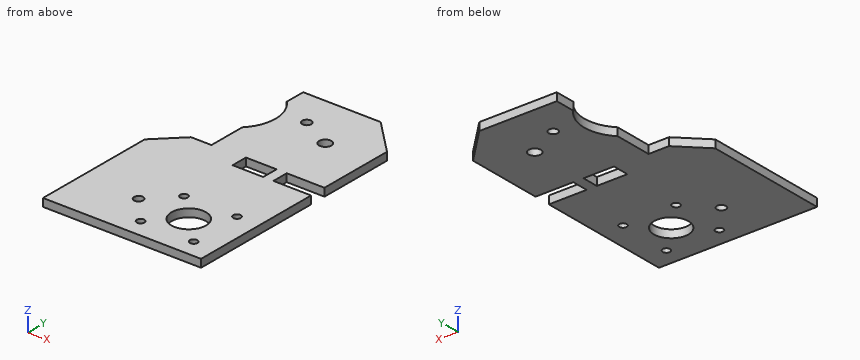
```python
from build123d import *

# Parameters (mm, degrees)
SKETCH1_W            = 155
SKETCH1_H            = 257
BOSS_EXTRUDE1_DEPTH  = 7.7
CHAMFER1_SIZE        = 34
SKETCH2_R            = 4.5
SKETCH2_W            = 37
SKETCH2_H            = 16
CUT_EXTRUDE1_DEPTH   = 10
SKETCH3_R            = 38.109899267
CUT_EXTRUDE2_DEPTH   = 10
CUT_EXTRUDE3_DEPTH   = 10
SKETCH5_R            = 16.935062279
CUT_EXTRUDE4_DEPTH   = 10
SKETCH6_R            = 3.705491154
CUT_EXTRUDE5_DEPTH   = 10
LPATTERN1_COUNT      = 2
LPATTERN1_PITCH      = 52
LPATTERN1_COUNT_DIR2 = 2
LPATTERN1_PITCH_DIR2 = 52
SKETCH7_R            = 6
CUT_EXTRUDE6_DEPTH   = 10
SKETCH8_W            = 30
SKETCH8_H            = 16
CUT_EXTRUDE7_DEPTH   = 10


with BuildPart() as part:
    # Sketch1 → Boss-Extrude1 (new body)
    with BuildSketch(Plane.XY):
        with Locations((64.176783005, -115.237481032)):
            Rectangle(SKETCH1_W, SKETCH1_H)
    extrude(amount=BOSS_EXTRUDE1_DEPTH)

    # Chamfer1
    chamfer1_edges = [part.edges().sort_by_distance(p)[0] for p in [
        (141.676783005, 13.262518968, 3.85),
    ]]
    chamfer(chamfer1_edges, length=CHAMFER1_SIZE)

    # Sketch2 → Cut-Extrude1 (cut)
    with BuildSketch(Plane.XY.offset(7.7)):
        with Locations((64.676783005, -22.737481032)):
            Circle(SKETCH2_R)
        with Locations((43.676783005, -198.737481032)):
            Circle(SKETCH2_R)
        with Locations((123.176783005, -103.737481032)):
            Rectangle(SKETCH2_W, SKETCH2_H)
    extrude(amount=-CUT_EXTRUDE1_DEPTH, mode=Mode.SUBTRACT)

    # Sketch3 → Cut-Extrude2 (cut)
    with BuildSketch(Plane.XY.offset(7.7)):
        with Locations((4.429117296, -33.119350325)):
            Circle(SKETCH3_R)
    extrude(amount=-CUT_EXTRUDE2_DEPTH, mode=Mode.SUBTRACT)

    # Sketch4 → Cut-Extrude3 (cut)
    with BuildSketch(Plane.XY.offset(7.7)):
        Polygon((31.676783005, 13.262518968), (31.676783005, -96.737481032), (11.676783005, -96.737481032), (-13.323216995, -121.737481032), (-67.69781948, -122.43585218), (-69.553853122, 22.073398829), (23.898503121, 29.809405578), align=None)
    extrude(amount=-CUT_EXTRUDE3_DEPTH, mode=Mode.SUBTRACT)

    # Sketch5 → Cut-Extrude4 (cut)
    with BuildSketch(Plane.XY.offset(7.7)):
        with Locations((93.676783005, -199.737481032)):
            Circle(SKETCH5_R)
    extrude(amount=-CUT_EXTRUDE4_DEPTH, mode=Mode.SUBTRACT)

    # Sketch6 → Cut-Extrude5 (cut)
    with BuildSketch(Plane.XY.offset(7.7)):
        with Locations((67.676783005, -225.737481032)):
            Circle(SKETCH6_R)
    cut_extrude5 = extrude(amount=-CUT_EXTRUDE5_DEPTH, mode=Mode.SUBTRACT)

    # LPattern1: Cut-Extrude5 2 × 2
    with Locations(*[(j * LPATTERN1_PITCH_DIR2, i * LPATTERN1_PITCH, 0) for i in range(LPATTERN1_COUNT) for j in range(LPATTERN1_COUNT_DIR2) if (i, j) != (0, 0)]):
        add(cut_extrude5, mode=Mode.SUBTRACT)

    # Sketch7 → Cut-Extrude6 (cut)
    with BuildSketch(Plane.XY.offset(7.7)):
        with Locations((96.676783005, -39.737481032)):
            Circle(SKETCH7_R)
    extrude(amount=-CUT_EXTRUDE6_DEPTH, mode=Mode.SUBTRACT)

    # Sketch8 → Cut-Extrude7 (cut)
    with BuildSketch(Plane.XY.offset(7.7)):
        with Locations((79.676783005, -103.737481032)):
            Rectangle(SKETCH8_W, SKETCH8_H)
    extrude(amount=-CUT_EXTRUDE7_DEPTH, mode=Mode.SUBTRACT)


solid = part.part
```
Geometry: final body of the model. Coordinates: model frame, mm. Coordinates: 2 decimals unless noted, no trailing zeros. Loops run counter-clockwise (first coordinate to the right, second up) from the corner with the lowest first, then second, coordinate; pieces in that order, holes last. Notation, with made-up numbers: (34, 44.25) -> (81, 44.25) arc R17 ccw to (81, 56.25) -> close; hole circle Ø2 at (35, -9.75). An arc over 180 degrees is marked (long way). Use a Markdown table: item, result. Add a question column.
(1) Section query B-B, the plane z = 3.25. State how many separate pieces and enclosed holes the cut face has, plus the area to 3 significant figures.
(2) Line query: line 1 along Y through (x, z) = (72.5, 1.25); line 2 along Y through (x, z) = (123, 3); line 3 along Y through (x, z) = (101, 5.5). Output: solid intervals per line, ascending.
(3) Section query C-C, the plane x = 36. Return loops of the section in (y, z).
(4) Pin query (flat end, axial travel): pin 1 Ø10.5 at (x, y) = (64.68, -22.74) entering from +Z; pin 2 Ø1.5 at (x, z) = (116.5, 3) entering from +Y; pin 3 Ø4 at (y, z) = (-1.5, 2.5) entering from -X. Return the tip coordinate at first contact, or that it passes through.
(5) Section query D-D, the plane x = 15. Return loops of the section in (y, z).
(6) Section query A-A, the plane x = 99.5. Return loops of the section in (y, z), plus the area to 3 significant figures.
Answer:
| question | item | result |
|---|---|---|
| 1 | separate pieces | 1 |
| 1 | enclosed holes | 9 |
| 1 | area | 31,200 mm^2 |
| 2 | line 1 | y = -243.74 to -111.74, -95.74 to 13.26 |
| 2 | line 2 | y = -243.74 to -227.38, -224.1 to -175.38, -172.1 to -111.74, -95.74 to -2.06 |
| 2 | line 3 | y = -243.74 to -215.01, -184.47 to -43.9, -35.58 to 13.26 |
| 3 | outline | (-243.74, 0) -> (-54.47, 0) -> (-54.47, 7.7) -> (-243.74, 7.7) -> close; (-11.77, 0) -> (13.26, 0) -> (13.26, 7.7) -> (-11.77, 7.7) -> close |
| 4 | pin 1 | stops at z = 7.7 |
| 4 | pin 2 | stops at y = 5.19 |
| 4 | pin 3 | stops at x = 31.68 |
| 5 | outline | (-243.74, 0) -> (-96.74, 0) -> (-96.74, 7.7) -> (-243.74, 7.7) -> close |
| 6 | outline | (-243.74, 0) -> (-215.64, 0) -> (-215.64, 7.7) -> (-243.74, 7.7) -> close; (-183.84, 0) -> (-45.03, 0) -> (-45.03, 7.7) -> (-183.84, 7.7) -> close; (-34.44, 0) -> (13.26, 0) -> (13.26, 7.7) -> (-34.44, 7.7) -> close |
| 6 | area | 1,650 mm^2 |
